Read the model definition and answer for the solid it produces. Units are mm, in the model's axes. Face numbers are marked on the shaded views. A direction names the side the tool comes from. Give positions to 0.01 mm unless a question says otherwise; leave off trailing zeros. Loops run counter-clockwise (first coordinate to the right, second up) from the corner with the lowest first, then second, coordinate; pieces in that order, holes last.
(1) Find section D-D, the plane y = 9.5. Write down the section's boundary in (x, z), then the cut area to 3 significant figures.
(2) Find section B-B, the plane z = 15. Write down the section's boundary in (x, y), then the cut area to 3 significant figures.
(3) Straight lines are drawn through the part: probe 1 along Z at (x, y) = (-3, 0); probe 2 along Z at (x, y) = (-9, 0); probe 3 along X at (y, z) = (4.5, 19.5). For each, find the intervals that lie inside material, in ascending order.
(4) Find section C-C, the plane y = 3.5. Write down the section's boundary in (x, z).
(5) Which of the six approach directions +Z, -Z, +X, -X, +Y, -Y give full straight-line access (tool end or side, diameter ignored) to the marked faces 5, 6 and 7?
(6) Each of these flat-tipped pins is pushed along its axis until it touches: P1, Ø9.5, axis at y = 12, z = 22, coming from the -X side; P2, Ø8, axis at x = -27.5, z = 12.5, coming from the -Y side; P3, Ø6, axis at y = 16, z = 17.5, coming from the +X side; P4, Ø3.5, axis at x = -27, z = 22.5, coming from the +Y side. Where does it stop, or does it pass through?
(7) Find section A-A, the plane x = -27. Write down the section's boundary in (y, z).
(8) Determine the mould class of the marked faces 1, 2, 3 and 4 for opening direction Y: pulls with the +Y half, pulls with the -Y half, needs draft (parallel to the pull), parting line crosses it, or undercut.
```python
from build123d import *

# Parameters (mm, degrees)
EXTRUDE_491_DEPTH      = 30
SKETCH_2_5_R           = 8.75
CUT_EXTRUDE_1383_DEPTH = 19
SKETCH_2_6_R           = 8.75
CUT_EXTRUDE_1659_DEPTH = 14
SKETCH_557_R           = 7.58383997
CUT_EXTRUDE_2951_DEPTH = 7
CUT_EXTRUDE_5_DEPTH    = 16.5
CUT_EXTRUDE_6_REACH    = 54.022
SKETCH_3_R             = 2.15


with BuildPart() as part:
    # Sketch 319 → Extrude 491 (new body)
    with BuildSketch(Plane.XY):
        Polygon((0, 18.75), (0, -18.75), (-22, -18.75), (-22, -3.75), (-34, -3.75), (-34, 6.75), (-22, 6.75), (-22, 18.75), align=None)
    extrude(amount=EXTRUDE_491_DEPTH)

    # Sketch 2_5 → Cut-Extrude 1383 (cut)
    with BuildSketch(Plane(origin=(0, 0, 0), x_dir=(0, 0, -1), z_dir=(1, 0, 0))):
        with Locations((-15, 0)):
            Circle(SKETCH_2_5_R)
    extrude(amount=-CUT_EXTRUDE_1383_DEPTH, mode=Mode.SUBTRACT)

    # Sketch 2_6 → Cut-Extrude 1659 (cut)
    with BuildSketch(Plane(origin=(0, 0, 0), x_dir=(0, 0, -1), z_dir=(1, 0, 0))):
        with BuildLine():
            Line((-7.139195711, 16.940201189), (-7.952107708, 18.75))
            Line((-7.952107708, 18.75), (-21.953209217, 18.75))
            Line((-21.953209217, 18.75), (-22.747558186, 16.94723086))
            Line((-22.747558186, 16.94723086), (-22.752278555, 5.746710121))
            ThreePointArc((-22.752278555, 5.746710121), (-15.008722765, -9.649996058), (-7.237345061, 5.732685958))
            Line((-7.237345061, 5.732685958), (-7.139195711, 16.940201189))
        make_face()
        with Locations((-15, 0)):
            Circle(SKETCH_2_6_R, mode=Mode.SUBTRACT)
    extrude(amount=-CUT_EXTRUDE_1659_DEPTH, mode=Mode.SUBTRACT)

    # Sketch 557 → Cut-Extrude 2951 (cut)
    with BuildSketch(Plane(origin=(0, 0, 0), x_dir=(0, 0, -1), z_dir=(1, 0, 0))):
        with BuildLine():
            Line((-22.752278555, 5.746710121), (-22.751322621, 8.014954624))
            ThreePointArc((-22.751322621, 8.014954624), (-19.352887132, -10.265226428), (-3.85, 0))
            ThreePointArc((-3.85, 0), (-4.726344075, 4.332954411), (-7.21762223, 7.984804083))
            Line((-7.21762223, 7.984804083), (-7.237345061, 5.732685958))
            ThreePointArc((-7.237345061, 5.732685958), (-5.833972503, 3.017687843), (-5.35, 0))
            ThreePointArc((-5.35, 0), (-18.025971906, -9.163296024), (-22.752278555, 5.746710121))
        make_face()
        with Locations((-15, 0)):
            Circle(SKETCH_557_R)
    extrude(amount=-CUT_EXTRUDE_2951_DEPTH, mode=Mode.SUBTRACT)

    # Sketch 7 → Cut-Extrude 5 (cut)
    with BuildSketch(Plane(origin=(0, 0, 0), x_dir=(0, 0, -1), z_dir=(1, 0, 0))):
        Polygon((-22.747558186, 16.94723086), (-22.750001382, 11.15), (-15, 11.15), (-7.189903158, 11.15), (-7.139195711, 16.940201189), (-7.952107708, 18.75), (-21.953209217, 18.75), align=None)
    extrude(amount=-CUT_EXTRUDE_5_DEPTH, mode=Mode.SUBTRACT)

    # Sketch 3 → Cut-Extrude 6 (cut, up to next)
    with BuildSketch(Plane(origin=(0, 6.75, 0), x_dir=(1, 0, 0), z_dir=(0, 1, 0)), mode=Mode.PRIVATE) as cut_extrude_6_sk1:
        with Locations(Location((-27, -7.5, 0), (0, 0, 270))):
            Circle(SKETCH_3_R)
    cut_extrude_6_tool1 = extrude(cut_extrude_6_sk1.sketch, amount=-CUT_EXTRUDE_6_REACH, mode=Mode.PRIVATE) & part.part
    # Sketch 3 → Cut-Extrude 6 (cut, up to next)
    with BuildSketch(Plane(origin=(0, 6.75, 0), x_dir=(1, 0, 0), z_dir=(0, 1, 0)), mode=Mode.PRIVATE) as cut_extrude_6_sk2:
        with Locations(Location((-27, -22.5, 0), (0, 0, 270))):
            Circle(SKETCH_3_R)
    cut_extrude_6_tool2 = extrude(cut_extrude_6_sk2.sketch, amount=-CUT_EXTRUDE_6_REACH, mode=Mode.PRIVATE) & part.part
    add(cut_extrude_6_tool1.solids().sort_by_distance((-27, 6.75, 7.5))[0], mode=Mode.SUBTRACT)
    add(cut_extrude_6_tool2.solids().sort_by_distance((-27, 6.75, 22.5))[0], mode=Mode.SUBTRACT)


solid = part.part
```
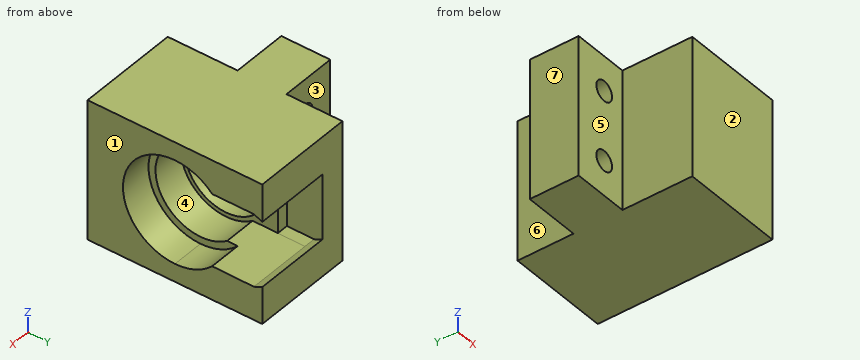
Entries:
1. outline: (-22, 0) - (0, 0) - (0, 7.2) - (-14, 7.2) - (-14, 22.75) - (0, 22.75) - (0, 30) - (-22, 30) - close
1. area: 442 mm2
2. outline: (-34, -3.75) - (-22, -3.75) - (-22, -18.75) - (0, -18.75) - (0, -11.15) - (-7, -11.15) - (-7, -9.65) - (-14, -9.65) - (-14, -8.75) - (-19, -8.75) - (-19, 8.75) - (-14, 8.75) - (-14, 11.15) - (-16.5, 11.15) - (-16.5, 18.75) - (-22, 18.75) - (-22, 6.75) - (-34, 6.75) - close
2. area: 436 mm2
3. probe 1: z = 0 to 3.85, 26.15 to 30
3. probe 2: z = 0 to 5.35, 24.65 to 30
3. probe 3: x = -34 to -19
4. outline: (-34, 0) - (0, 0) - (0, 4.41) - (-7, 4.41) - (-7, 6.01) - (-14, 6.01) - (-14, 6.98) - (-19, 6.98) - (-19, 23.02) - (-14, 23.02) - (-14, 23.99) - (-7, 23.99) - (-7, 25.59) - (0, 25.59) - (0, 30) - (-34, 30) - close; hole circle Ø4.3 at (-27, 7.5); hole circle Ø4.3 at (-27, 22.5)
5. face 5: +Z, -Z, -X, -Y
5. face 6: +Z, -Z, -X, +Y
5. face 7: +Z, -Z, -X, +Y, -Y
6. P1: stops at x = -22
6. P2: stops at y = -3.75
6. P3: stops at x = -16.5
6. P4: passes through
7. outline: (-3.75, 0) - (6.75, 0) - (6.75, 5.35) - (-3.75, 5.35) - close; (-3.75, 9.65) - (6.75, 9.65) - (6.75, 20.35) - (-3.75, 20.35) - close; (-3.75, 24.65) - (6.75, 24.65) - (6.75, 30) - (-3.75, 30) - close
8. face 1: needs draft
8. face 2: pulls with the -Y half
8. face 3: pulls with the +Y half
8. face 4: undercut
